Here's how the part is built. I have some questions about the finished solid (model axes, mm). A direction names the side the tool comes from. Round coordinates to 2 decimals unless told otherwise and drop trailing zeros. Order: outer loops, then holes, each group sorted by start corner. A loop starts at its lowest first (then second) coordinate and runs counter-clockwise, first axis right, second up. Notation, with made-up numbers: (24, -1.5) - (67, -1.5) arc R8 ccw to (67, 13.5) - close; hole circle Ø2 at (26, -37.75). An arc over 180 degrees is marked (long way). One line per item, written item: value.
from build123d import *

# Parameters (mm, degrees)
SKETCH1_W           = 81.28
SKETCH1_H           = 55.626
BOSS_EXTRUDE1_DEPTH = 2.54
SKETCH2_W           = 2.54
SKETCH2_H           = 18.499605323
SKETCH2_H_2         = 18.818048641
CUT_EXTRUDE1_DEPTH  = 50.311501387
CAVITY9_START       = -27.813
CAVITY9_OUTLINE_W   = 27.093333334
CAVITY9_OUTLINE_H   = 2.54
CAVITY9_DEPTH       = 2.54
CAVITY9_START_2     = 25.273
CAVITY9_2_OUTLINE_W = 27.093333334
CAVITY9_2_OUTLINE_H = 2.54
CAVITY9_2_DEPTH     = 2.54


# Read off the part's stored shape, not the designer's step: Cavity9
with BuildPart() as part:
    # Sketch1 → Boss-Extrude1 (new body)
    with BuildSketch(Plane.XY):
        Rectangle(SKETCH1_W, SKETCH1_H)
    extrude(amount=BOSS_EXTRUDE1_DEPTH)

    # Sketch2 → Cut-Extrude1 (cut, through all)
    with BuildSketch(Plane.XY.offset(2.54)):
        with Locations((-39.37, 18.563197339)):
            Rectangle(SKETCH2_W, SKETCH2_H)
        with Locations((-39.37, -18.595234966)):
            Rectangle(SKETCH2_W, SKETCH2_H_2)
        with Locations((39.469570783, -18.595234966)):
            Rectangle(SKETCH2_W, SKETCH2_H_2)
        with Locations((39.469570783, 18.563197339)):
            Rectangle(SKETCH2_W, SKETCH2_H)
    extrude(amount=-CUT_EXTRUDE1_DEPTH, mode=Mode.SUBTRACT)

    # Cavity9 outline → Cavity9 (cut)
    with BuildSketch(Plane(origin=(0, 0, 0), x_dir=(1, 0, 0), z_dir=(0, 1, 0)).offset(CAVITY9_START)):
        with Locations((0, -1.27)):
            Rectangle(CAVITY9_OUTLINE_W, CAVITY9_OUTLINE_H)
    extrude(amount=CAVITY9_DEPTH, mode=Mode.SUBTRACT)

    # Cavity9 2 outline → Cavity9 2 (cut)
    with BuildSketch(Plane(origin=(0, 0, 0), x_dir=(1, 0, 0), z_dir=(0, 1, 0)).offset(CAVITY9_START_2)):
        with Locations((0, -1.27)):
            Rectangle(CAVITY9_2_OUTLINE_W, CAVITY9_2_OUTLINE_H)
    extrude(amount=CAVITY9_2_DEPTH, mode=Mode.SUBTRACT)


solid = part.part
Q1. If we section it at A-A, the plane z = 1.35: Please give me the cut outline in (x, y), then the cut area to 3 significant figures.
Results list:
outline: (-40.64, -9.19) - (-38.1, -9.19) - (-38.1, -27.81) - (-13.55, -27.81) - (-13.55, -25.27) - (13.55, -25.27) - (13.55, -27.81) - (38.2, -27.81) - (38.2, -9.19) - (40.64, -9.19) - (40.64, 9.31) - (38.2, 9.31) - (38.2, 27.81) - (13.55, 27.81) - (13.55, 25.27) - (-13.55, 25.27) - (-13.55, 27.81) - (-38.1, 27.81) - (-38.1, 9.31) - (-40.64, 9.31) - close
area: 4,200 mm²
Q2. Will these pins go through, and if not, where does the flat tip stop? pin 1 (0.8 mm diameter, centred on x = 5.5, z = 1, fed in from +Y); pin 2 (1.3 mm diameter, centred on x = -1.5, z = 1, fed in from -Y); pin 3 (0.8 mm diameter, centred on x = -39.5, z = 1, fed in from +Y).
Results list:
pin 1: y = 25.27
pin 2: y = -25.27
pin 3: y = 9.31
Q3. We'd pull the mould along X, two halves only. Please class faces 1 (the flat face through (-39, -9.186, 1)), 2 (the flat face through (38.2, 18, 1)), 3 (the flat face through (0, 25.273, 1)): released by +X, released by -X, zero draft, split by the parting line, or undercut.
Results list:
face 1: zero draft
face 2: released by +X
face 3: undercut
Q4. If we section it at B-B, the plane y = -20.5: Please give me the cut outline in (x, z), then the cut area to 3 significant figures.
Results list:
outline: (-38.1, 0) - (38.2, 0) - (38.2, 2.54) - (-38.1, 2.54) - close
area: 194 mm²
Q5. If we section it at C-C, the plane x = 0: Please give me the cut outline in (y, z).
Results list:
outline: (-25.27, 0) - (25.27, 0) - (25.27, 2.54) - (-25.27, 2.54) - close
Q6. If I drill on line 1 along X through (y, z) = (19.5, 1), over which ranges is the centre line in solid material (lowest first)?
Results list:
line 1: -38.1 to 38.2
Q7. Which directions (+Z, -Z, +X, -X, +Y, -Y) give clear straight access to the entire face, cutting with the end or side of a thin tool? Please do faces 4 (the flat face through (13.547, -27, 1)), 5 (the flat face through (13.547, 27, 1)), 6 (the flat face through (38.2, -19, 1)), 7 (the flat face through (39, 9.313, 1)).
Results list:
face 4: +Z, -Z, -Y
face 5: +Z, -Z, +Y
face 6: +Z, -Z, +X, -Y
face 7: +Z, -Z, +X, +Y
